Input: dimensioned drawing with shaded views. Units: mm. Origin: part minimum x, y, z. Give positions to 0.01 mm unless a question says otherwise; leave off trailing zeros. Order: outer loops, then holes, each group sorted by start corner. A loop starts at its lowest first (then second) coordinate and runs counter-clockwise, first axis right, second up. Notation, with made-up numbers: M 83.5,23 L 117.5,23 A20 ccw 117.5,54 Z; hole C 71,65 d3. An arc over 180 degrees is marked long. Answer in a Markdown table with one row per item. Add a question column.
(1) Pin query (flat end, axial travel): P1, Ø5, axis at x = 10, y = 75, coming from the -Z side. Return the tip coordinate at first contact, or that it passes through.
(2) Material intervals for line 1 along X through (y, z) = (59, 1.8) (1 decimal); line 2 along Y through (x, z) = (10, 1.8); line 3 along Y through (x, z) = (84, 1.75), sorted ascending.
(3) Section query D-D, the plane x = 66. Return loops of the section in (y, z).
(4) Section query A-A, the plane y = 75. Return loops of the section in (x, z).
(5) Section query C-C, the plane y = 135. Return loops of the section in (x, z), plus the area to 3 significant figures.
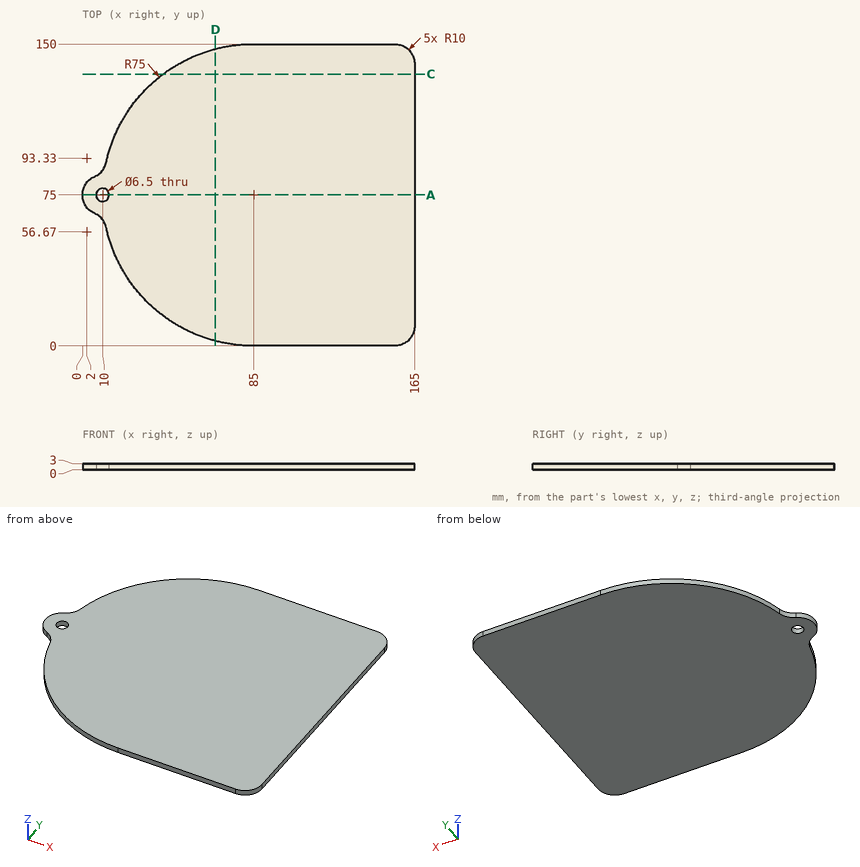
Values follow:
| question | item | result |
|---|---|---|
| 1 | P1 | passes through |
| 2 | line 1 | x = 11.7 to 165 |
| 2 | line 2 | y = 62.67 to 71.75, 78.25 to 87.33 |
| 2 | line 3 | y = 0.01 to 149.99 |
| 3 | outline | M 2.45,0 L 147.55,0 L 147.55,3 L 2.45,3 Z |
| 4 | outline | M 0,0 L 6.75,0 L 6.75,3 L 0,3 Z; M 13.25,0 L 165,0 L 165,3 L 13.25,3 Z |
| 5 | outline | M 40,0 L 165,0 L 165,3 L 40,3 Z |
| 5 | area | 375 mm² |
